Work out the finished part from the listing and answer in its coordinate system (mm). A direction names the side the tool comes from. Round coordinates to 2 decimals unless told otherwise and drop trailing zeros. Order: outer loops, then holes, each group sorted by start corner. A loop starts at its lowest first (then second) coordinate and runs counter-clockwise, first axis right, second up. Notation, with made-up numbers: (20.5, 20) - (34.5, 20) arc R22 ccw to (34.5, 58) - close; hole circle Ø4 at (-39.5, -37). An arc over 180 degrees is marked (long way). One line per question, with ' | ' between items. Start each with the question number.
from build123d import *

# Parameters (mm, degrees)
F0_R     = 304.8
F0_R_2   = 48.006
F1_DEPTH = 12.7
F3_DEPTH = 12.701
F4_R     = 5.08


with BuildPart() as f1:
    # F0 (on Front) → F1 (new body)
    with BuildSketch(Plane.XZ):
        Circle(F0_R)
        Circle(F0_R_2, mode=Mode.SUBTRACT)
    extrude(amount=F1_DEPTH)

    # F2 (on face) → F3 (cut, through all)
    with BuildSketch(Plane.XZ.offset(12.7)):
        with BuildLine():
            Line((-25.4, 232.156), (-25.4, 130.556))
            ThreePointArc((-25.4, 130.556), (0, 105.156), (25.4, 130.556))
            Line((25.4, 130.556), (25.4, 232.156))
            ThreePointArc((25.4, 232.156), (0, 257.556), (-25.4, 232.156))
        make_face()
        with BuildLine():
            Line((188.352994, 138.075045), (100.364813, 87.275045))
            ThreePointArc((100.364813, 87.275045), (91.067767, 52.578), (125.764813, 43.280955))
            Line((125.764813, 43.280955), (213.752994, 94.080955))
            ThreePointArc((213.752994, 94.080955), (223.050039, 128.778), (188.352994, 138.075045))
        make_face()
        with BuildLine():
            Line((213.752994, -94.080955), (125.764813, -43.280955))
            ThreePointArc((125.764813, -43.280955), (91.067767, -52.578), (100.364813, -87.275045))
            Line((100.364813, -87.275045), (188.352994, -138.075045))
            ThreePointArc((188.352994, -138.075045), (223.050039, -128.778), (213.752994, -94.080955))
        make_face()
        with BuildLine():
            Line((25.4, -232.156), (25.4, -130.556))
            ThreePointArc((25.4, -130.556), (0, -105.156), (-25.4, -130.556))
            Line((-25.4, -130.556), (-25.4, -232.156))
            ThreePointArc((-25.4, -232.156), (0, -257.556), (25.4, -232.156))
        make_face()
        with BuildLine():
            Line((-188.352994, -138.075045), (-100.364813, -87.275045))
            ThreePointArc((-100.364813, -87.275045), (-91.067767, -52.578), (-125.764813, -43.280955))
            Line((-125.764813, -43.280955), (-213.752994, -94.080955))
            ThreePointArc((-213.752994, -94.080955), (-223.050039, -128.778), (-188.352994, -138.075045))
        make_face()
        with BuildLine():
            Line((-213.752994, 94.080955), (-125.764813, 43.280955))
            ThreePointArc((-125.764813, 43.280955), (-91.067767, 52.578), (-100.364813, 87.275045))
            Line((-100.364813, 87.275045), (-188.352994, 138.075045))
            ThreePointArc((-188.352994, 138.075045), (-223.050039, 128.778), (-213.752994, 94.080955))
        make_face()
    extrude(amount=-F3_DEPTH, mode=Mode.SUBTRACT)

    # F4
    f4_edges = [f1.edges().sort_by_distance(p)[0] for p in [
        (-304.8, 0, 0),
        (-304.8, -12.7, 0),
    ]]
    fillet(f4_edges, radius=F4_R)


solid = f1.part
1) Section A-A on x = 0 is taken. Give the vertices of the cut face in (y, z), and give its area (3 significant figures).
2) Straight lines are drawn through the part: line 1 (Z direction, x = 0, y = -6.5); line 2 (Z direction, x = -219.5, y = -8.25); line 3 (X direction, y = -10.25, z = 52). For each, find the intervals that lie inside material, in ascending order.
3) For faces 4 (the cylindrical face through (-0.559, -6.439, 105.162)), 5 (the flat face through (-4, -12.7, -62)), determine the directions among +Z, -Z, +X, -X, +Y, -Y from which every point of the face is accessible in a straight line to the end or side of a thin tool.
4) Flat-ended cylindrical pins translate along their axes: pin 1 (1 mm diameter, centred on y = -5, z = -94, fed in from +X); pin 2 (5 mm diameter, centred on x = -217.5, z = 101.5, fed in from +Y); pin 3 (3 mm diameter, centred on y = -10.5, z = -67, fed in from -X); pin 4 (4 mm diameter, centred on y = -7.5, z = 195.5, fed in from -X). Find the tip coordinate at first contact, or state that the pin passes through.
5) Section C-C on x = -152 is taken. Give the number of separate pieces and of enclosed holes in the cut face, and give its area (3 significant figures).
6) Determine the mould class of faces 1 (the flat face through (-4, 0, -62)), 2 (the cylindrical face through (-241.879, -6.332, -185.466)), 3 (the cylindrical face through (0.56, -6.44, 257.55)) for opening direction X: released by +X, released by -X, zero draft, split by the parting line, or undercut.
7) Section B-B on z = 0 is taken. Give the vertices of the cut face in (x, y).
Recorded:
1) outline: (-12.7, -299.72) arc R5.08 ccw to (-7.62, -304.8) - (-5.08, -304.8) arc R5.08 ccw to (0, -299.72) - (0, -257.56) - (-12.7, -257.56) - close; (-12.7, -105.16) - (0, -105.16) - (0, -48.01) - (-12.7, -48.01) - close; (-12.7, 48.01) - (0, 48.01) - (0, 105.16) - (-12.7, 105.16) - close; (-12.7, 257.56) - (0, 257.56) - (0, 299.72) arc R5.08 ccw to (-5.08, 304.8) - (-7.62, 304.8) arc R5.08 ccw to (-12.7, 299.72) - close | area: 2,630 mm²
2) line 1: z = -304.8 to -257.56, -105.16 to -48.01, 48.01 to 105.16, 257.56 to 304.8 | line 2: z = -211.42 to -133.54, -98.62 to 98.62, 133.54 to 211.42 | line 3: x = -299.59 to -140.87, -91.41 to 91.41, 140.87 to 299.59
3) face 4: +Y, -Y | face 5: +Z, -Z, +X, -X, -Y
4) pin 1: stops at x = 290.1 | pin 2: passes through | pin 3: stops at x = -297.26 | pin 4: stops at x = -235.5
5) separate pieces: 3 | enclosed holes: 0 | area: 5,200 mm²
6) face 1: zero draft | face 2: split by the parting line | face 3: undercut
7) outline: (-304.8, -7.62) arc R5.08 ccw to (-299.72, -12.7) - (-48.01, -12.7) - (-48.01, 0) - (-299.72, 0) arc R5.08 ccw to (-304.8, -5.08) - close; (48.01, -12.7) - (299.72, -12.7) arc R5.08 ccw to (304.8, -7.62) - (304.8, -5.08) arc R5.08 ccw to (299.72, 0) - (48.01, 0) - close
